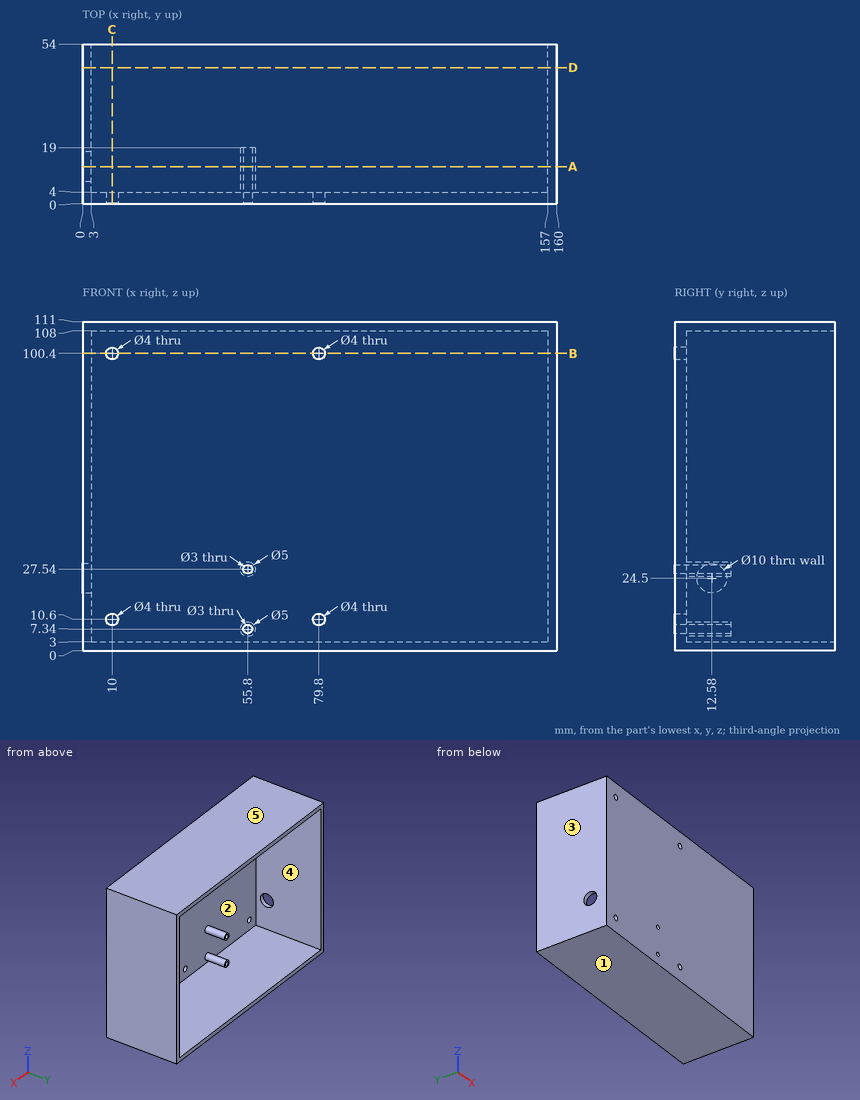
Source: three-view drawing plus pictorial views. Frame: mm from the lowest corner of the part. A direction names the side the tool comes from. Round coordinates to 2 decimals unless told otherwise and drop trailing zeros. Order: outer loops, then holes, each group sorted by start corner. A loop starts at its lowest first (then second) coordinate and runs counter-clockwise, first axis right, second up. Notation, with made-up numbers: (41.25, -40) -> (56.25, -40) arc R21 cw to (56.25, -21) -> close; hole circle Ø10 at (73, -34.75). An arc over 180 degrees is marked (long way). Use CSV: the item, a comma, the result in double quotes. Start each with the question number.
1) First-contact query: pin 1 Ø2.5 at (x, z) = (55, 27) entering from +Y; pin 2 Ø5 at (x, z) = (24.5, 87.5) entering from +Y. Flat tips, straight axial feed; report the tip coordinate or a pass-through.
2) Set-up query: the marked faces 1 and 2. Return all of +Z, -Z, +X, -X, +Y, -Y with unobstructed straight access to the full face (end or side cutting, diameter ignored); none if empty.
3) Section D-D (y = 46). Return the cut outline in (x, z), and give its area (3 significant figures).
4) Draft query along Z for the marked faces 3, 4 and 5. Return one class per face: +Z half, -Z half, draft (parallel to the pull), parting line (faces both ways), or undercut.
5) Section A-A (y = 12.58). Return the cut outline in (x, z).
6) Section B-B (z = 100.4). Return the cut outline in (x, y).
7) Section C-C (x = 10). Return the cut outline in (y, z), and give its area (3 significant figures).
8) Material intervals for line 1 along X through (y, z) = (1.3, 100.4); line 2 along Y through (x, z) = (1.05, 24.5); line 3 along Z through (x, y) = (117.5, 37), sorted ascending. Write a range as from..to.
Returned:
1,pin 1,"stops at y = 19"
1,pin 2,"stops at y = 4"
2,face 1,"-Z, +X, -X, +Y, -Y"
2,face 2,"+Y"
3,outline,"(0, 0) -> (160, 0) -> (160, 111) -> (0, 111) -> close; hole (3, 3) -> (157, 3) -> (157, 108) -> (3, 108) -> close"
3,area,"1,590 mm²"
4,face 3,"draft"
4,face 4,"undercut"
4,face 5,"+Z half"
5,outline,"(0, 0) -> (160, 0) -> (160, 111) -> (0, 111) -> (0, 29.5) -> (3, 29.5) -> (3, 108) -> (157, 108) -> (157, 3) -> (3, 3) -> (3, 19.5) -> (0, 19.5) -> close; circle Ø5 at (55.8, 7.34); circle Ø5 at (55.8, 27.54); hole circle Ø3 at (55.8, 7.34); hole circle Ø3 at (55.8, 27.54)"
6,outline,"(0, 0) -> (8, 0) -> (8, 4) -> (3, 4) -> (3, 54) -> (0, 54) -> close; (12, 0) -> (77.8, 0) -> (77.8, 4) -> (12, 4) -> close; (81.8, 0) -> (160, 0) -> (160, 54) -> (157, 54) -> (157, 4) -> (81.8, 4) -> close"
7,outline,"(0, 0) -> (54, 0) -> (54, 3) -> (4, 3) -> (4, 8.6) -> (0, 8.6) -> close; (0, 12.6) -> (4, 12.6) -> (4, 98.4) -> (0, 98.4) -> close; (0, 102.4) -> (4, 102.4) -> (4, 108) -> (54, 108) -> (54, 111) -> (0, 111) -> close"
7,area,"712 mm²"
8,line 1,"x = 0..8, 12..77.8, 81.8..160"
8,line 2,"y = 0..7.58, 17.58..54"
8,line 3,"z = 0..3, 108..111"
